For this review, take the finished solid that the model builds, in its own axes (mm). Coordinates: 2 decimals unless noted, no trailing zeros. Write each loop counter-clockwise with the first axis right and the second up, starting at its lowest first coordinate (ties: lowest second). Pieces come first, ordered by that corner, then holes. Notation, with made-up numbers: M -39.5,84.5 L -13.5,84.5 A33 cw -13.5,119.5 Z; hole C -38,-9 d1. An arc over 180 degrees is marked long. One line per question, with ' | ' between items.
Autodesk Inventor part; units mm, degrees
ref_plane "YZ Plane" through (0, 0, 0) normal (1, 0, 0) x (0, 1, 0)
ref_plane "XZ Plane" through (0, 0, 0) normal (0, 1, 0) x (-1, 0, 0)
ref_plane "XY Plane" through (0, 0, 0) normal (0, 0, 1) x (1, 0, 0)
ref_plane "Work Plane1" through (0, 0, 0) normal (0, 0, 1) x (1, 0, 0)
sketch "Sketch1" plane through (228.6, 0, 0) normal (0, 0, -1) x (-1, 0, 0)
  circle A0 centre (-12.7, 0) radius 2.1971
  circle A1 centre (114.3, 0) radius 2.1971
  circle A2 centre (-12.7, 76.2) radius 2.1971
  circle A3 centre (114.3, 76.2) radius 2.1971
  line L0 (-17.78, 120.65) -> (119.38, 120.65)
  line L1 (119.38, 120.65) -> (119.38, -12.7)
  line L2 (119.38, -12.7) -> (-17.78, -12.7)
  line L3 (-17.78, -12.7) -> (-17.78, 120.65)
  circle A4 centre (114.3, 114.3) radius 2.1844
  circle A5 centre (-12.7, 114.3) radius 2.1844
  point P0 (228.6, 0)
  dimension "d0" = 12.7
  dimension "d2" = 5.08
  dimension "d3" = 5.08
  dimension "d6" = 6.35
extrude "Extrusion1" add sketch "Sketch1" along normal blind 1.5
fillet "Fillet2" radius 5.715 4 edges at (246.38, 120.65, -0.75) (109.22, 120.65, -0.75) (109.22, -12.7, -0.75) (246.38, -12.7, -0.75)
sketch "Sketch7" plane through (109.22, -6.985, 0) normal (-1, 0, 0) x (0, 0, 1)
  circle A0 centre (-9.3619, 102.3193) radius 2.2479
  arc A1 (-12.6628, 105.7523) -> (-12.0724, 98.4034) centre (-9.3619, 102.3193) ccw
  line L0 (-12.6628, 105.7523) -> (-1.5, 116.4856)
  line L1 (-12.0724, 98.4034) -> (-1.5, 91.0856)
  line L2 (-1.5, 0) -> (-1.5, 121.92)
  point P0 (0, 6.985)
  dimension "d38" = 9.525
  dimension "d39" = 25.4
  dimension "d40" = 78.566
extrude "Extrusion6" add sketch "Sketch7" against normal up to surface (137.16 mm away)
sketch "Sketch8" plane through (228.6, 0, -1.5) normal (0, 0, -1) x (-1, 0, 0)
  arc A0 (-17.78, -6.985) -> (-12.065, -12.7) centre (-12.065, -6.985) ccw
  line L0 (-17.78, 114.935) -> (-17.78, -6.985)
  arc A1 (-12.065, 120.65) -> (-17.78, 114.935) centre (-12.065, 114.935) ccw
  line L1 (113.665, 120.65) -> (-12.065, 120.65)
  arc A2 (119.38, 114.935) -> (113.665, 120.65) centre (113.665, 114.935) ccw
  line L2 (119.38, -6.985) -> (119.38, 114.935)
  arc A3 (113.665, -12.7) -> (119.38, -6.985) centre (113.665, -6.985) ccw
  line L3 (-12.065, -12.7) -> (113.665, -12.7)
  circle A4 centre (-12.7, 114.3) radius 2.1844
  circle A5 centre (114.3, 114.3) radius 2.1844
  circle A6 centre (114.3, 76.2) radius 2.1971
  circle A7 centre (-12.7, 76.2) radius 2.1971
  circle A8 centre (114.3, 0) radius 2.1971
  circle A9 centre (-12.7, 0) radius 2.1971
  line L4 (119.38, 84.1006) -> (-17.78, 84.1006)
  line L5 (-17.78, 109.5006) -> (119.38, 109.5006)
  line L6 (-12.7, 109.5006) -> (-12.7, 84.1006)
  line L7 (114.3, 84.1006) -> (114.3, 109.5006)
  point P0 (228.6, 0)
  dimension "d43" = 5.08
  dimension "d44" = 5.08
extrude "Extrusion7" cut sketch "Sketch8" along normal through all contours L6 L5 L7 L4
chamfer "Chamfer2" distance 3.175 angle 45 2 edges at (114.3, 96.8006, -1.5) (241.3, 96.8006, -1.5)
sketch "Sketch9" plane through (228.6, 0, -1.5) normal (0, 0, -1) x (-1, 0, 0)
  line L0 (113.665, 120.65) -> (-12.065, 120.65)
  line L1 (-6.35, 120.65) -> (107.95, 120.65)
  line L2 (107.95, 120.65) -> (107.95, 82.55)
  line L3 (107.95, 82.55) -> (-6.35, 82.55)
  line L4 (-6.35, 82.55) -> (-6.35, 120.65)
  line L5 (119.38, -6.985) -> (119.38, 84.1006)
  line L6 (-17.78, 84.1006) -> (-17.78, -6.985)
  point P0 (228.6, 0)
  dimension "d50" = 38.1
  dimension "d51" = 114.3
  dimension "d52" = 11.43
  dimension "d53" = 11.43
extrude "Extrusion8" cut sketch "Sketch9" against normal through all
fillet "Fillet3" radius 5.715 4 edges at (234.95, 82.55, -0.75) (120.65, 82.55, -0.75) (120.65, 120.65, -0.75) (234.95, 120.65, -0.75)
equation "\"d52\" = d53"
properties part number "bottom rails" material "Acetal Resin, Black"
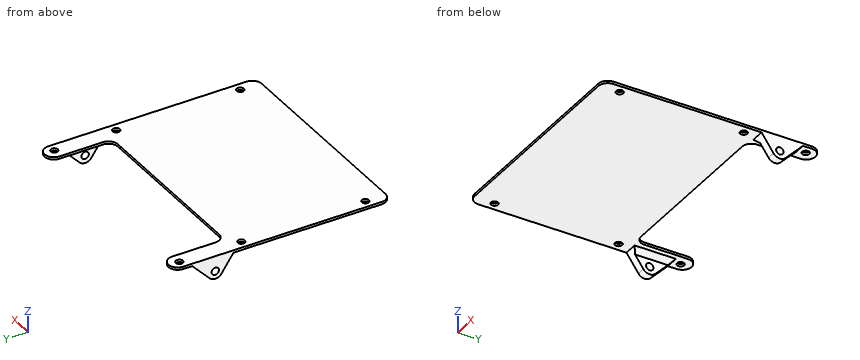
1. Take a section at B-B on x = 157.5. State the section outline as (y, z) points.
Computed values:
outline: M -12.7,-1.5 L 82.55,-1.5 L 82.55,0 L -12.7,0 Z
2. For line 1 along Y through (x, z) = (241.3, -0.55); line 2 along Z through (x, y) = (191, 67); line 3 along Y through (x, z) = (122, -0.75), list the stretches that pass through material, from the lowest coordinate up.
Computed values:
line 1: y = -12.66 to -2.2, 2.2 to 74, 78.4 to 112.12, 116.48 to 120.61 | line 2: z = -1.5 to 0 | line 3: y = -12.7 to 84.58
3. Take a section at A-A on y = 76.2. State the section outline as (x, z) points.
Computed values:
outline: M 109.22,-1.5 L 112.1,-1.5 L 112.1,0 L 109.22,0 Z; M 116.5,-1.5 L 239.1,-1.5 L 239.1,0 L 116.5,0 Z; M 243.5,-1.5 L 246.38,-1.5 L 246.38,0 L 243.5,0 Z
4. Clearance check with flat-ended pins moving along their axes: P1, Ø5.5, axis at x = 114.3, y = 76.2, coming from the -Z side; P2, Ø5, axis at y = 95.33, z = -9.36, coming from the -X side; P3, Ø1.2, axis at x = 195.5, z = -0.5, coming from the +Y side. State where each tip first meets the part, or that it passes through.
Computed values:
P1: stops at z = -1.5 | P2: stops at x = 109.22 | P3: stops at y = 82.55
